```python
from build123d import *

# Parameters (mm, degrees)
SKETCH1_W           = 10
SKETCH1_H           = 9.875
BOSS_EXTRUDE1_DEPTH = 240
SKETCH2_W           = 9.875
SKETCH2_H           = 10
BOSS_EXTRUDE2_DEPTH = 20
SKETCH3_R           = 1.5
CUT_EXTRUDE1_DEPTH  = 242.349081014
FILLET1_R           = 5


with BuildPart() as part:
    # Sketch1 → Boss-Extrude1 (new body)
    with BuildSketch(Plane(origin=(0, 0, 0), x_dir=(1, 0, 0), z_dir=(0, 1, 0))):
        Rectangle(SKETCH1_W, SKETCH1_H)
    extrude(amount=BOSS_EXTRUDE1_DEPTH)

    # Sketch2 → Boss-Extrude2 (add)
    with BuildSketch(Plane(origin=(5, 0, 0), x_dir=(0, 0, -1), z_dir=(1, 0, 0))):
        with Locations((0, 5)):
            Rectangle(SKETCH2_W, SKETCH2_H)
        with Locations((0, 235)):
            Rectangle(SKETCH2_W, SKETCH2_H)
    extrude(amount=BOSS_EXTRUDE2_DEPTH)

    # Sketch3 → Cut-Extrude1 (cut, through all)
    with BuildSketch(Plane(origin=(0, 240, 0), x_dir=(1, 0, 0), z_dir=(0, 1, 0))):
        with Locations(Location((10, 0, 0), (0, 0, 270))):
            Circle(SKETCH3_R)
        with Locations(Location((20, 0, 0), (0, 0, 270))):
            Circle(SKETCH3_R)
    extrude(amount=-CUT_EXTRUDE1_DEPTH, mode=Mode.SUBTRACT)

    # Fillet1
    # the kernel refuses this fillet: 5 mm, written as the material it adds along each edge
    with BuildSketch(Plane(origin=(5, 10, 4.9375), x_dir=(0, 1, 0), z_dir=(0, 0, -1))) as fillet1_piece_1_section:
        with BuildLine():
            CenterArc((FILLET1_R, FILLET1_R), FILLET1_R, 180, 90)
            Line((0, FILLET1_R), (0, 0))
            Line((0, 0), (FILLET1_R, 0))
        make_face()
    fillet1_piece_1 = extrude(amount=9.875, mode=Mode.PRIVATE)
    fillet1_piece_1 = fillet1_piece_1 - Plane(origin=(10, 11.142134011, 0), x_dir=(0, 0, 1), z_dir=(0, 1, 0)) * Cylinder(1.5, 40, mode=Mode.PRIVATE)
    add(fillet1_piece_1)
    with BuildSketch(Plane(origin=(5, 230, 4.9375), x_dir=(1, 0, 0), z_dir=(0, 0, -1))) as fillet1_piece_2_section:
        with BuildLine():
            CenterArc((FILLET1_R, FILLET1_R), FILLET1_R, 180, 90)
            Line((0, FILLET1_R), (0, 0))
            Line((0, 0), (FILLET1_R, 0))
        make_face()
    fillet1_piece_2 = extrude(amount=9.875, mode=Mode.PRIVATE)
    fillet1_piece_2 = fillet1_piece_2 - Plane(origin=(10, 228.857865929, 0), x_dir=(0, 0, 1), z_dir=(0, 1, 0)) * Cylinder(1.5, 40, mode=Mode.PRIVATE)
    add(fillet1_piece_2)


solid = part.part
```
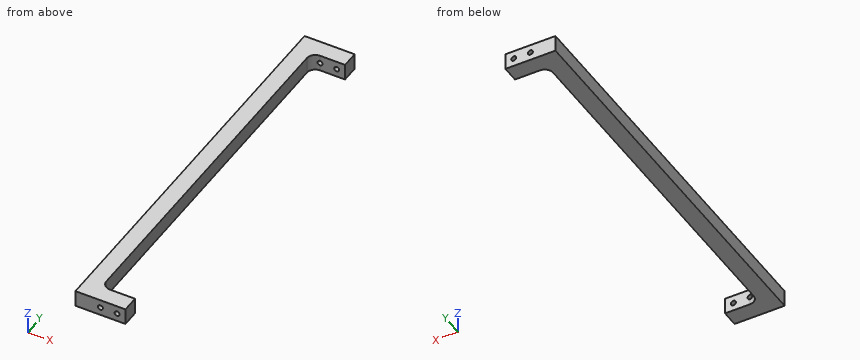
Design review of the part built by this model. Coordinates are the model's own, in mm. Coordinates: 2 decimals unless noted, no trailing zeros. Loops run counter-clockwise (first coordinate to the right, second up) from the corner with the lowest first, then second, coordinate; pieces in that order, holes last. Notation, with made-up numbers: (-3.75, -2) - (53.25, -2) arc R26 cw to (53.25, 24) - close; hole circle Ø5 at (-18.75, -22). An arc over 180 degrees is marked (long way). Use CSV: the item, a comma, the result in double quotes. Start each with the question number.
1) For pin 1 Ø3 at (y, z) = (186, 3) entering from +X, flat-tipped, find the tip position at first contact; note if it passes through.
2) Consider section B-B on y = 147.5. Write out the cut boundary in (x, z).
3) Wall thickness on L1, parallel to X at y = 3.25, z = 0; L2, parallel to Y at x = 15.5, z = 1.25; L3, parallel to Z at x = 10, y = 4: over which ranges is each line inside the solid? List them lowest first. Write a range as from..to.
4) Consider section A-A on z = 0. Write out the cut boundary in (x, y), then the cut area to 3 significant figures.
Geometry says:
1,pin 1,"x = 5"
2,outline,"(-5, -4.94) - (5, -4.94) - (5, 4.94) - (-5, 4.94) - close"
3,L1,"-5..8.5, 11.5..18.5, 21.5..25"
3,L2,"0..10, 230..240"
3,L3,"-4.94..-1.5, 1.5..4.94"
4,outline,"(-5, 0) - (8.5, 0) - (8.5, 10.23) arc R5 cw to (5, 15) - (5, 225) arc R5 cw to (8.5, 229.77) - (8.5, 240) - (-5, 240) - close; (11.5, 0) - (18.5, 0) - (18.5, 10) - (11.5, 10) - close; (11.5, 230) - (18.5, 230) - (18.5, 240) - (11.5, 240) - close; (21.5, 0) - (25, 0) - (25, 10) - (21.5, 10) - close; (21.5, 230) - (25, 230) - (25, 240) - (21.5, 240) - close"
4,area,"2,690 mm^2"
